Geometry check sheet. Reference: the model listing, model coordinates, mm. A direction names the side the tool comes from. Round coordinates to 2 decimals unless told otherwise and drop trailing zeros. Order: outer loops, then holes, each group sorted by start corner. A loop starts at its lowest first (then second) coordinate and runs counter-clockwise, first axis right, second up. Notation, with made-up numbers: (74.25, 3) - (122.25, 3) arc R28 cw to (122.25, 41) - close; hole circle Ø5 at (-23, 88). An arc over 180 degrees is marked (long way). One line per question, with ' | ' between items. Start each with the question number.
Q1. Sectioned sample at C-C, the plane z = -14.5. Enter the section's corners in (x, y), then the cut area to 3 significant figures.
Q2. Sectioned sample at A-A, the plane z = -7. Enter the section's corners in (x, y).
Q3. Mould release check, pull along X, two halves, no side actions. Record for faces 3 (the face through (11.2, 18, -5)), 4 (the face through (15, 6, 0)), 5 (the face through (19.5, 20.64, -9.41)): +X half, -X half, draft (parallel to the pull), parting line (faces both ways), or undercut.
Q4. Material ranges on line 1 along Y through (x, z) = (16.25, -1); line 2 along Z through (x, y) = (2, 7); line 3 along Y through (x, z) = (2.75, -4.5), recorded low to high.
Q5. Sectioned sample at B-B, the plane y = 4.5. Enter the section's corners in (x, z), then the cut area to 3 significant figures.
Q6. Sectioned sample at D-D, the plane x = 5.75. Enter the section's corners in (y, z).
Q7. Tool access check on faces 1 (the face through (14.479, 6.544, -4.93)), 2 (the face through (5, 16, 0)). Record the directions out of +Z, -Z, +X, -X, +Y, -Y that give a thin tool (end or side, any length) a straight path to the whole face; none if there is none.
```python
from build123d import *

# Parameters (mm, degrees)
SKETCH1_W       = 20.4
SKETCH1_H       = 21.5
EXTRUDE1_DEPTH  = 16
EXTRUDE10_DEPTH = 10
FILLET8_R       = 3


with BuildPart() as part:
    # Sketch1 → Extrude1 (new body)
    with BuildSketch(Plane.XY):
        with Locations((10.2, 10.75)):
            Rectangle(SKETCH1_W, SKETCH1_H)
    extrude(amount=-EXTRUDE1_DEPTH)

    # Sketch11 → Extrude10 (cut)
    with BuildSketch(Plane.XY):
        with BuildLine():
            Line((2, 11.75), (4.283920217, 11.75))
            ThreePointArc((4.283920217, 11.75), (5.957359313, 14.992640687), (9.2, 16.666079783))
            Line((9.2, 16.666079783), (9.2, 19.5))
            ThreePointArc((9.2, 19.5), (10.2, 20.5), (11.2, 19.5))
            Line((11.2, 19.5), (11.2, 16.666079783))
            ThreePointArc((11.2, 16.666079783), (14.442640687, 14.992640687), (16.116079783, 11.75))
            Line((16.116079783, 11.75), (18.4, 11.75))
            ThreePointArc((18.4, 11.75), (19.4, 10.75), (18.4, 9.75))
            Line((18.4, 9.75), (16.116079783, 9.75))
            ThreePointArc((16.116079783, 9.75), (14.442640687, 6.507359313), (11.2, 4.833920217))
            Line((11.2, 4.833920217), (11.2, 2))
            ThreePointArc((11.2, 2), (10.2, 1), (9.2, 2))
            Line((9.2, 2), (9.2, 4.833920217))
            ThreePointArc((9.2, 4.833920217), (5.957359313, 6.507359313), (4.283920217, 9.75))
            Line((4.283920217, 9.75), (2, 9.75))
            ThreePointArc((2, 9.75), (1, 10.75), (2, 11.75))
        make_face()
    extrude(amount=-EXTRUDE10_DEPTH, mode=Mode.SUBTRACT)

    # Fillet8
    # the kernel refuses this fillet: 3 mm, written as the material it takes off along each edge
    with BuildSketch(Plane(origin=(17.4, 3, -3), x_dir=(1, 0, 0), z_dir=(0, -1, 0))) as fillet8_piece_1_section:
        Polygon((0, 0), (FILLET8_R, 0), (FILLET8_R, FILLET8_R), (0, FILLET8_R), align=None)
    fillet8_piece_1 = extrude(amount=FILLET8_R, mode=Mode.PRIVATE)
    fillet8_piece_1 = fillet8_piece_1 - Plane(origin=(17.4, 3, -3), x_dir=(-0.7071067811865475, 0, -0.7071067811865475), z_dir=(0, -1, 0)) * Sphere(FILLET8_R, mode=Mode.PRIVATE)
    add(fillet8_piece_1, mode=Mode.SUBTRACT)
    with BuildSketch(Plane(origin=(17.4, 18.5, -3), x_dir=(0, 0, 1), z_dir=(1, 0, 0))) as fillet8_piece_2_section:
        Polygon((0, 0), (FILLET8_R, 0), (FILLET8_R, -FILLET8_R), (0, -FILLET8_R), align=None)
    fillet8_piece_2 = extrude(amount=FILLET8_R, mode=Mode.PRIVATE)
    fillet8_piece_2 = fillet8_piece_2 - Plane(origin=(17.4, 18.5, -3), x_dir=(0, -0.7071067811865475, -0.7071067811865475), z_dir=(1, 0, 0)) * Sphere(FILLET8_R, mode=Mode.PRIVATE)
    add(fillet8_piece_2, mode=Mode.SUBTRACT)
    with BuildSketch(Plane(origin=(3, 3, -3), x_dir=(-1, 0, 0), z_dir=(0, -1, 0))) as fillet8_piece_3_section:
        Polygon((0, 0), (FILLET8_R, 0), (FILLET8_R, -FILLET8_R), (0, -FILLET8_R), align=None)
    fillet8_piece_3 = extrude(amount=FILLET8_R, mode=Mode.PRIVATE)
    fillet8_piece_3 = fillet8_piece_3 - Plane(origin=(3, 3, -3), x_dir=(0.7071067811865475, 0, -0.7071067811865475), z_dir=(0, -1, 0)) * Sphere(FILLET8_R, mode=Mode.PRIVATE)
    add(fillet8_piece_3, mode=Mode.SUBTRACT)
    with BuildSketch(Plane(origin=(3, 18.5, -3), x_dir=(0, 0, 1), z_dir=(-1, 0, 0))) as fillet8_piece_4_section:
        Polygon((0, 0), (FILLET8_R, 0), (FILLET8_R, FILLET8_R), (0, FILLET8_R), align=None)
    fillet8_piece_4 = extrude(amount=FILLET8_R, mode=Mode.PRIVATE)
    fillet8_piece_4 = fillet8_piece_4 - Plane(origin=(3, 18.5, -3), x_dir=(0, -0.7071067811865475, -0.7071067811865475), z_dir=(-1, 0, 0)) * Sphere(FILLET8_R, mode=Mode.PRIVATE)
    add(fillet8_piece_4, mode=Mode.SUBTRACT)
    with BuildSketch(Plane(origin=(20.4, 3, 0), x_dir=(0, 0, -1), z_dir=(0, 1, 0)), Plane(origin=(0, 18.5, 0), x_dir=(0, 0, -1), z_dir=(0, -1, 0))) as fillet8_piece_5:
        with BuildLine():
            CenterArc((FILLET8_R, FILLET8_R), FILLET8_R, 180, 90)
            Line((0, FILLET8_R), (0, 0))
            Line((0, 0), (FILLET8_R, 0))
        make_face()
    extrude(amount=15.5, mode=Mode.SUBTRACT)
    with BuildSketch(Plane(origin=(3, 0, 0), x_dir=(0, 0, -1), z_dir=(1, 0, 0))) as fillet8_piece_6:
        with BuildLine():
            CenterArc((FILLET8_R, FILLET8_R), FILLET8_R, 180, 90)
            Line((0, FILLET8_R), (0, 0))
            Line((0, 0), (FILLET8_R, 0))
        make_face()
    extrude(amount=14.4, mode=Mode.SUBTRACT)
    with BuildSketch(Plane(origin=(17.4, 21.5, 0), x_dir=(0, -1, 0), z_dir=(-1, 0, 0))) as fillet8_piece_7:
        with BuildLine():
            CenterArc((FILLET8_R, -FILLET8_R), FILLET8_R, 90, 90)
            Line((0, -FILLET8_R), (0, 0))
            Line((0, 0), (FILLET8_R, 0))
        make_face()
    extrude(amount=14.4, mode=Mode.SUBTRACT)
    with BuildSketch(Plane(origin=(20.4, 0, -3), x_dir=(-1, 0, 0), z_dir=(0, 0, -1)), Plane(origin=(20.4, 21.5, -3), x_dir=(0, -1, 0), z_dir=(0, 0, -1))) as fillet8_piece_8:
        with BuildLine():
            CenterArc((FILLET8_R, FILLET8_R), FILLET8_R, 180, 90)
            Line((0, FILLET8_R), (0, 0))
            Line((0, 0), (FILLET8_R, 0))
        make_face()
    extrude(amount=20.5, mode=Mode.SUBTRACT)
    with BuildSketch(Plane(origin=(0, 21.5, -3), x_dir=(0, -1, 0), z_dir=(0, 0, -1)), Plane(origin=(0, 0, -3), x_dir=(1, 0, 0), z_dir=(0, 0, -1))) as fillet8_piece_9:
        with BuildLine():
            CenterArc((FILLET8_R, -FILLET8_R), FILLET8_R, 90, 90)
            Line((0, -FILLET8_R), (0, 0))
            Line((0, 0), (FILLET8_R, 0))
        make_face()
    extrude(amount=20.5, mode=Mode.SUBTRACT)


solid = part.part
```
Determined:
1) outline: (0, 3) arc R3 ccw to (3, 0) - (17.4, 0) arc R3 ccw to (20.4, 3) - (20.4, 18.5) arc R3 ccw to (17.4, 21.5) - (3, 21.5) arc R3 ccw to (0, 18.5) - close | area: 431 mm2
2) outline: (0, 3) arc R3 ccw to (3, 0) - (17.4, 0) arc R3 ccw to (20.4, 3) - (20.4, 18.5) arc R3 ccw to (17.4, 21.5) - (3, 21.5) arc R3 ccw to (0, 18.5) - close; hole (2, 9.75) - (4.28, 9.75) arc R6 ccw to (9.2, 4.83) - (9.2, 2) arc R1 ccw to (11.2, 2) - (11.2, 4.83) arc R6 ccw to (16.12, 9.75) - (18.4, 9.75) arc R1 ccw to (18.4, 11.75) - (16.12, 11.75) arc R6 ccw to (11.2, 16.67) - (11.2, 19.5) arc R1 ccw to (9.2, 19.5) - (9.2, 16.67) arc R6 ccw to (4.28, 11.75) - (2, 11.75) arc R1 ccw to start
3) face 3: undercut | face 4: draft | face 5: +X half
4) line 1: y = 0.76 to 9.75, 11.75 to 20.74 | line 2: z = -16 to -0.17 | line 3: y = 0.01 to 9.75, 11.75 to 21.49
5) outline: (0, -16) - (20.4, -16) - (20.4, -3) arc R3 ccw to (17.4, 0) - (11.2, 0) - (11.2, -10) - (9.2, -10) - (9.2, 0) - (3, 0) arc R3 ccw to (0, -3) - close | area: 303 mm2
6) outline: (0, -16) - (21.5, -16) - (21.5, -3) arc R3 ccw to (18.5, 0) - (14.77, 0) - (14.77, -10) - (6.73, -10) - (6.73, 0) - (3, 0) arc R3 ccw to (0, -3) - close
7) face 1: +Z | face 2: +Z, +X, -X, +Y, -Y
